Could you check a few things on this drawing? It's one solid part, dimensions in mm from its lowest x, y, z. A direction names the side the tool comes from. Round coordinates to 2 decimals unless told otherwise and drop trailing zeros. Write each loop counter-clockwise with the first axis right and the second up, starting at its lowest first coordinate (ties: lowest second). Pieces come first, ordered by that corner, then holes. Notation, with made-up numbers: (37, -10) - (94, -10) arc R19 ccw to (94, 19) - close; hole circle Ø11 at (61.5, 12.25). An arc over 180 degrees is marked (long way). Put each result on its own line as item: value.
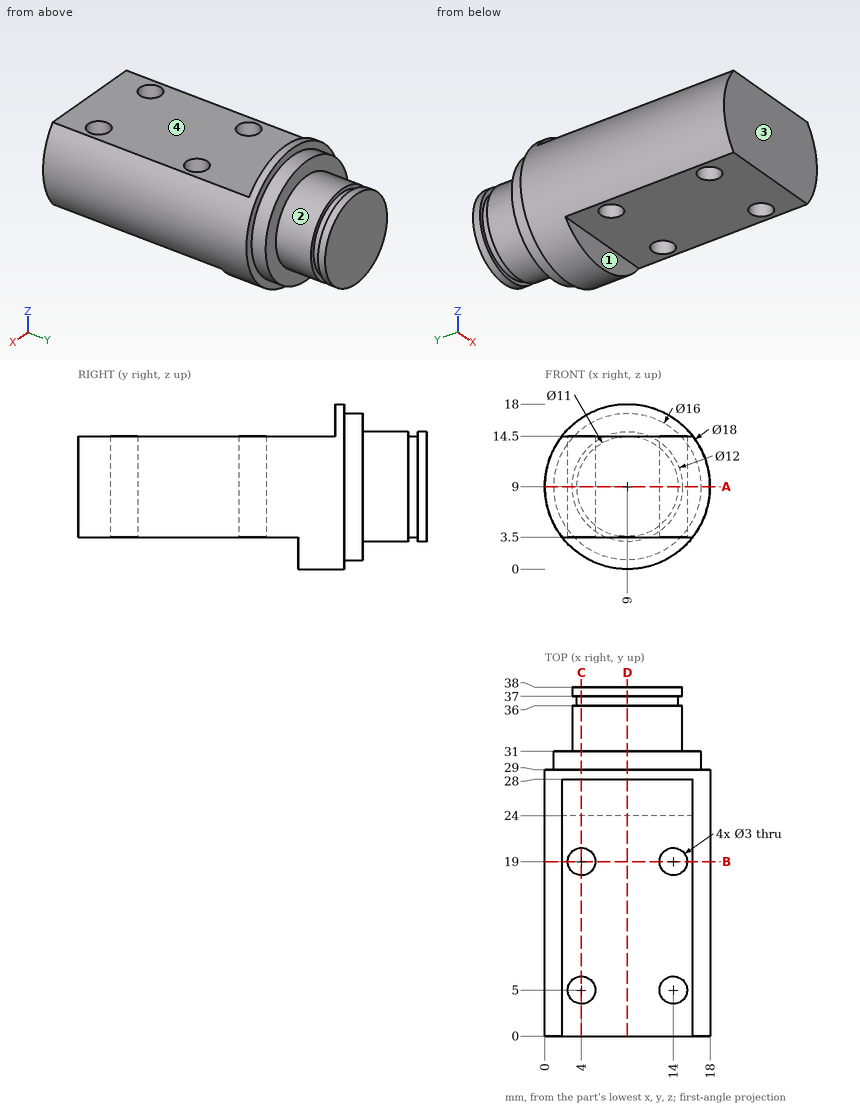
(1) I'm going to push flat-ended pins straight in: pin 1 (3 mm diameter, centred on x = 7.5, z = 17, fed in from -Y); pin 2 (3 mm diameter, centred on x = 9.5, y = 33.5, fed in from -Z); pin 3 (2 mm diameter, centred on y = 20.5, z = 12, fed in from +X); pin 4 (1.8 mm diameter, centred on x = 14, y = 19, fed in from -Z). Where does each tip first touch, or does it pass through?
Values found:
pin 1: stops at y = 28
pin 2: stops at z = 3
pin 3: stops at x = 17.77
pin 4: passes through
(2) Please list where these lines run through material, in increasing order: probe 1 along Y at (x, z) = (14, 9.75); probe 2 along Y at (x, z) = (4, 12); probe 3 along Y at (x, z) = (2.75, 12). Write a range as from..to.
Values found:
probe 1: y = 0..3.5, 6.5..17.5, 20.5..38
probe 2: y = 0..3.5, 6.5..17.5, 20.5..36, 37..38
probe 3: y = 0..4.17, 5.83..18.17, 19.83..31
(3) Imagine slicing it at B-B, the plane y = 19. List the corners of the cut face in (x, z) for me, then the cut area to 3 significant figures.
Values found:
outline: (1.88, 3.5) - (2.5, 3.5) - (2.5, 14.5) - (1.88, 14.5) arc R9 ccw to start; (5.5, 3.5) - (12.5, 3.5) - (12.5, 14.5) - (5.5, 14.5) - close; (15.5, 3.5) - (16.12, 3.5) arc R9 ccw to (16.12, 14.5) - (15.5, 14.5) - close
area: 119 mm^2
(4) For the marked faces 1, 2, 3 and 4, which set-ups out of +Z, -Z, +X, -X, +Y, -Y let a thin tool reach every point of the face, with its end or its side?
Values found:
face 1: -Z, +X, -X, -Y
face 2: +Y
face 3: +Z, -Z, +X, -X, -Y
face 4: +Z, +X, -X, -Y
(5) Imagine slicing it at D-D, the plane x = 9. List the corners of the cut face in (y, z) for me.
Values found:
outline: (0, 3.5) - (24, 3.5) - (24, 0) - (29, 0) - (29, 1) - (31, 1) - (31, 3) - (36, 3) - (36, 3.5) - (37, 3.5) - (37, 3) - (38, 3) - (38, 15) - (37, 15) - (37, 14.5) - (36, 14.5) - (36, 15) - (31, 15) - (31, 17) - (29, 17) - (29, 18) - (28, 18) - (28, 14.5) - (0, 14.5) - close
(6) Imagine slicing it at A-A, the plane z = 9. List the corners of the cut face in (x, y) for me, then the cut area to 3 significant figures.
Values found:
outline: (0, 0) - (18, 0) - (18, 29) - (17, 29) - (17, 31) - (15, 31) - (15, 36) - (14.5, 36) - (14.5, 37) - (15, 37) - (15, 38) - (3, 38) - (3, 37) - (3.5, 37) - (3.5, 36) - (3, 36) - (3, 31) - (1, 31) - (1, 29) - (0, 29) - close; hole circle Ø3 at (4, 5); hole circle Ø3 at (4, 19); hole circle Ø3 at (14, 5); hole circle Ø3 at (14, 19)
area: 609 mm^2
(7) Imagine slicing it at C-C, the plane x = 4. Give the number of separate pieces and of enclosed holes in the cut face, then the cut area to 3 significant figures.
Values found:
separate pieces: 3
enclosed holes: 0
area: 334 mm^2
